Autodesk Inventor part; units mm, degrees
ref_plane "YZ Plane" through (0, 0, 0) normal (1, 0, 0) x (0, 1, 0)
ref_plane "XZ Plane" through (0, 0, 0) normal (0, 1, 0) x (-1, 0, 0)
ref_plane "XY Plane" through (0, 0, 0) normal (0, 0, 1) x (1, 0, 0)
sketch "Sketch1" plane through (0, 0, 0) normal (0, 1, 0) x (-1, 0, 0)
  line L0 (4.8, 0) -> (-0.8, 0) construction
  line L1 (0, -37.7337) -> (0, 68.9023) construction
  line L2 (4, 22.5) -> (0, 22.5)
  line L3 (0, 22.5) -> (0, -22.5)
  line L4 (0, -22.5) -> (4, -22.5)
  line L5 (4, -22.5) -> (4, 22.5)
  line L6 (4, 53.6686) -> (4, 38.3314)
  line L7 (1.9878, -22.5) -> (4, 0.5)
  point P0 (0, 0)
  point P1 (0, 22.5)
  point P2 (0, -22.5)
  dimension "d2" = 8
  dimension "d5" = 23
  dimension "d21" = 45
  dimension "d22" = 3.9755
  dimension "d23" = 5
revolve "Revolution1" add sketch "Sketch1" angle 360 about axis through (0, 0, -10) along (0, 0, 1) contours L5 L7 L4 L3 L2
sketch "Sketch2" plane through (0, 0, 22.5) normal (0, 0, 1) x (1, 0, 0)
  circle A0 centre (0, 0) radius 4
hole "Hole1" at (0, 0, 22.5) direction (0, 0, -1) diameter 3.242 depth 25 tip angle 118
chamfer "Chamfer1" distance 0.5 angle 45 2 edges at (4, 0, 22.5) (0, 1.621, 22.5)
properties part number "DLT-01-238B" material "Poliacetal WT"
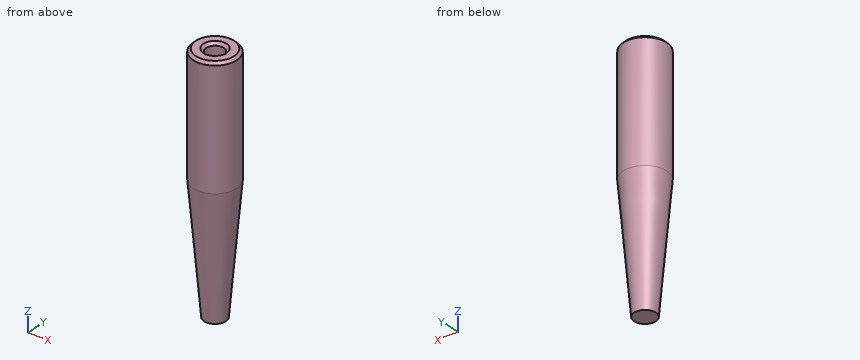
Can you work these out from the model? Positions are in its coordinate system, mm. Round coordinates to 2 decimals unless told otherwise and drop trailing zeros. Loops run counter-clockwise (first coordinate to the right, second up) from the corner with the lowest first, then second, coordinate; pieces in that order, holes last. Notation, with made-up numbers: (10.5, 44) -> (45.5, 44) arc R22 ccw to (45.5, 63) -> close; hole circle Ø5 at (74.25, 0). An arc over 180 degrees is marked (long way). Answer in a Markdown table with one row per item.
Item 1: Suppose I cut it at A-A, the plane z = 1.5. List the corners of the cut face in (x, y) for me.
Answer block:
| item | result |
|---|---|
| outline | circle Ø8 at (0, 0); hole circle Ø3.24 at (0, 0) |
Item 2: If I drill on probe 1 along Y at (x, z) = (0, 2.5); probe 2 along X at (y, z) = (-0.75, 1.5), over which ranges is the centre line in solid material (lowest first)?
Answer block:
| item | result |
|---|---|
| probe 1 | -4 to -1.62, 1.62 to 4 |
| probe 2 | -3.93 to -1.44, 1.44 to 3.93 |
Item 3: Will these pins go through, and if not, where does the flat tip stop? P1, Ø1, axis at x = -0.5, z = 0, coming from the +Y side; P2, Ø2, axis at x = 0.5, z = -3, coming from the -Y side; P3, Ø1, axis at y = 2, z = -0.5, coming from the -X side.
Answer block:
| item | result |
|---|---|
| P1 | y = 3.99 |
| P2 | y = -3.77 |
| P3 | x = -3.62 |
